from build123d import *

# Parameters (mm, degrees)
CYLINDER001_R       = 2
CYLINDER001_DEPTH   = 10
CYLINDER_W          = 20
CYLINDER_H          = 5
CYLINDER_ANGLE      = 270
CUT_PLACEMENT_ANGLE = 45


with BuildPart() as cilindro001:
    # Cylinder001 → Cylinder001 (new body)
    with BuildSketch(Plane(origin=(5, 10, 0), x_dir=(1, 0, 0), z_dir=(0, 0, 1))):
        Circle(CYLINDER001_R)
    extrude(amount=CYLINDER001_DEPTH)


with BuildPart() as cut:
    # Cylinder → Cylinder (revolve)
    with BuildSketch(Plane.XZ):
        with Locations((10, 2.5)):
            Rectangle(CYLINDER_W, CYLINDER_H)
    revolve(axis=Axis((0, 0, 0), (0, 0, 1)), revolution_arc=CYLINDER_ANGLE)

    # Cut: cut Cilindro001
    add(cilindro001.part, mode=Mode.SUBTRACT)


with BuildPart() as cut_1:
    # Cut placement: moved
    add(cut.part.rotate(Axis((0, 0, 0), (0, 0, 1)), CUT_PLACEMENT_ANGLE))


solid = cut_1.part
Build history of the part. All positions in model axes, mm. A direction names the side the tool comes from. Coordinates: 2 decimals unless noted, no trailing zeros. Order: outer loops, then holes, each group sorted by start corner. A loop starts at its lowest first (then second) coordinate and runs counter-clockwise, first axis right, second up. Notation, with made-up numbers: (21.25, -38.5) - (39.25, -38.5) arc R26 cw to (39.25, -5.5) - close; hole circle Ø9 at (-3, -32.5). An arc over 180 degrees is marked (long way). Write each question's results on one line, items separated by ' | '. Start each with the question number.
Item 1: Mould opens along X. For faces 3 (the face through (-5.011, 9.256, 2.465)), 4 (the face through (-6, 0, 5)), 5 (the face through (7, 7, 3)), 6 (the face through (-19.99, 0.66, 2.54)) say: released by +X, released by -X, zero draft, split by the parting line, or undercut.
Item 2: Band-saw the part on A-A on z = 0.85. Write the cut outline in (x, y), and give its area (3 significant figures).
Item 3: Flat gauge pins, fed straight in: pin 1 (1.5 mm diameter, centred on x = 10, z = 0.5, fed in from -Y); pin 2 (1.5 mm diameter, centred on y = 7.5, z = 1.5, fed in from -X); pin 3 (1 mm diameter, centred on y = 7, z = 2.5, fed in from -X); pin 4 (8 mm diameter, centred on x = 10, y = 9, fed in from -Z). Where does each tip first touch, or does it go through?
Item 4: Wall check: probe 1 along X at (y, z) = (10.5, 0.8); probe 2 along X at (y, z) = (11, 4.35); probe 3 along Y at (x, z) = (9.5, 1). Give the ranges that are in metal, low to high. Write a range as [from, to].
Item 5: Tool access for faces 1 (the face through (-6, 0, 0)), 2 (the face through (7, -7, 3)): list every direction of +Z, -Z, +X, -X, +Y, -Y with a clear straight run to the whole face (end or side of a thin tool).
Item 6: Band-saw the part on C-C on x = -11.5. Write the cut outline in (y, z), and give its area (3 significant figures).
Item 7: Band-saw the part on B-B on y = -7. Write the cut outline in (x, z) (3 decimals), and give its area (3 significant figures).
Numbers:
1) face 3: undercut | face 4: zero draft | face 5: released by +X | face 6: split by the parting line
2) outline: (0, 0) - (14.14, 14.14) arc R20 ccw (long way) to (14.14, -14.14) - close; hole circle Ø4 at (-3.54, 10.61) | area: 930 mm^2
3) pin 1: y = -17.73 | pin 2: x = -18.83 | pin 3: x = -18.91 | pin 4: z = 0
4) probe 1: [-17.02, -5.53], [-1.54, 10.5] | probe 2: [-16.7, -5.5], [-1.57, 11] | probe 3: [-17.6, -9.5], [9.5, 17.6]
5) face 1: -Z, +X, -X, +Y, -Y | face 2: +Z, -Z, +X
6) outline: (-16.36, 0) - (16.36, 0) - (16.36, 5) - (-16.36, 5) - close | area: 164 mm^2
7) outline: (-18.735, 0) - (7, 0) - (7, 5) - (-18.735, 5) - close | area: 129 mm^2
